```python
from build123d import *

# Parameters (mm, degrees)
SKETCH1_W               = 25
SKETCH1_H               = 3
BOSS_EXTRUDE1_DEPTH     = 288
SKETCH2_W               = 14
SKETCH2_H               = 20
SKETCH2_W_2             = 10
SKETCH2_H_2             = 16
BOSS_EXTRUDE2_DEPTH     = 18
CUT_EXTRUDE1_DEPTH      = 290.317299863
CUT_EXTRUDE1_DEPTH_BACK = 290.317299863
SKETCH3_R               = 2.5
SKETCH4_W               = 30
SKETCH4_H               = 50
BOSS_EXTRUDE3_DEPTH     = 2
BOSS_EXTRUDE4_DEPTH     = 7
FILLET1_R               = 1
SKETCH6_R               = 2.5
CUT_EXTRUDE2_DEPTH      = 10


with BuildPart() as part:
    # Sketch1 → Boss-Extrude1 (new body)
    with BuildSketch(Plane(origin=(0, 0, 0), x_dir=(1, 0, 0), z_dir=(0, 1, 0))):
        Rectangle(SKETCH1_W, SKETCH1_H)
    extrude(amount=BOSS_EXTRUDE1_DEPTH)

    # Sketch2 → Boss-Extrude2 (add)
    with BuildSketch(Plane.XY.offset(1.5)):
        with Locations((0, 278)):
            Rectangle(SKETCH2_W, SKETCH2_H)
        with Locations((0, 278)):
            Rectangle(SKETCH2_W_2, SKETCH2_H_2, mode=Mode.SUBTRACT)
    extrude(amount=BOSS_EXTRUDE2_DEPTH)

    # Sketch3 → Cut-Extrude1 (cut, two sides: drawn at the far end of the back side and taken through both)
    with BuildSketch(Plane.ZY.offset(7).offset(-CUT_EXTRUDE1_DEPTH_BACK)):
        with Locations(Location((6.5, 278, 0), (0, 0, 180))):
            Circle(SKETCH3_R)
    extrude(amount=CUT_EXTRUDE1_DEPTH + CUT_EXTRUDE1_DEPTH_BACK, mode=Mode.SUBTRACT)

    # Sketch4 → Boss-Extrude3 (add)
    with BuildSketch(Plane(origin=(0, 0, 0), x_dir=(-1, 0, 0), z_dir=(0, -1, 0))):
        Rectangle(SKETCH4_W, SKETCH4_H)
    extrude(amount=BOSS_EXTRUDE3_DEPTH)

    # Sketch5 → Boss-Extrude4 (add)
    with BuildSketch(Plane.XY.offset(1.5)):
        Polygon((0, 0), (1, 0), (1, 268), (0, 268), (-1, 268), (-1, 0), align=None)
    extrude(amount=BOSS_EXTRUDE4_DEPTH)

    # Fillet1
    fillet1_edges = [part.edges().sort_by_distance(p)[0] for p in [
        (-12.5, 288, 0),
        (9.75, 288, 1.5),
        (-9.75, 288, 1.5),
        (7, 278, 19.5),
        (0, 288, 19.5),
        (-7, 278, 19.5),
        (0, 268, 19.5),
        (7, 278, 1.5),
        (7, 268, 10.5),
        (7, 288, 10.5),
        (-7, 278, 1.5),
        (-7, 288, 10.5),
        (-4, 268, 1.5),
        (-7, 268, 10.5),
        (4, 268, 1.5),
        (1, 134, 1.5),
        (1, 268, 5),
        (-1, 134, 1.5),
        (-1, 268, 5),
        (1, 134, 8.5),
        (0, 268, 8.5),
        (-1, 134, 8.5),
        (0, 288, -1.5),
    ]]
    fillet(fillet1_edges, radius=FILLET1_R - 0.0001)  # a hair under: the kernel refuses the full size

    # Sketch6 → Cut-Extrude2 (cut)
    with BuildSketch(Plane(origin=(0, 0, 0), x_dir=(1, 0, 0), z_dir=(0, 1, 0))):
        with Locations(Location((8, 18, 0), (0, 0, 270))):
            Circle(SKETCH6_R)
        with Locations(Location((-8, 18, 0), (0, 0, 270))):
            Circle(SKETCH6_R)
        with Locations(Location((-8, -18, 0), (0, 0, 270))):
            Circle(SKETCH6_R)
        with Locations(Location((8, -18, 0), (0, 0, 270))):
            Circle(SKETCH6_R)
    extrude(amount=-CUT_EXTRUDE2_DEPTH, mode=Mode.SUBTRACT)


solid = part.part
```
The model under review builds one solid part; all positions refer to its coordinate system, in mm. A direction names the side the tool comes from. Give positions to 0.01 mm unless a question says otherwise; leave off trailing zeros. Write each loop counter-clockwise with the first axis right and the second up, starting at its lowest first coordinate (ties: lowest second). Pieces come first, ordered by that corner, then holes. Notation, with made-up numbers: M -11,16 L -5,16 A19 ccw -5,41 Z; hole C 51.25,7.5 d3. An arc over 180 degrees is marked long. Answer in a Markdown table with one row per item.
Item 1: Add section A-A on z = -18. Give the boundary of the cut face in (x, y), plus the area to 3 significant figures.
Check sheet entries:
| item | result |
|---|---|
| outline | M -15,-2 L -10.5,-2 L -10.5,0 L -15,0 Z; M -5.5,-2 L 5.5,-2 L 5.5,0 L -5.5,0 Z; M 10.5,-2 L 15,-2 L 15,0 L 10.5,0 Z |
| area | 40.0 mm2 |
Item 2: Add section B-B on y = 278. Give the boundary of the cut face in (x, z), plus the area to 3 significant figures.
Check sheet entries:
| item | result |
|---|---|
| outline | M -12.5,-1.5 L 12.5,-1.5 L 12.5,1.5 L 8,1.5 A1 cw 7,2.5 L 7,4 L 5,4 L 5,1.5 L -5,1.5 L -5,4 L -7,4 L -7,2.5 A1 cw -8,1.5 L -12.5,1.5 Z; M -7,9 L -5,9 L -5,19.5 L -6,19.5 A1 ccw -7,18.5 Z; M 5,9 L 7,9 L 7,18.5 A1 ccw 6,19.5 L 5,19.5 Z |
| area | 127 mm2 |
Item 3: For P1, Ø6, axis at x = 0, y = 274, coming from the +Z side; P2, Ø1.5, axis at x = -2, z = -9.5, coming from the +Y side; P3, Ø6.5, axis at x = -8, z = 18, coming from the -Y side; P4, Ø6.5, axis at y = 278, z = 6.5, coming from the +X side, all flat-tipped, find the tip position at first contact; note any pin that passes through.
Check sheet entries:
| item | result |
|---|---|
| P1 | z = 1.5 |
| P2 | y = 0 |
| P3 | y = -2 |
| P4 | x = 7 |
Item 4: For line 1 along X through (y, z) = (-1.2, -18); line 2 along Y through (x, z) = (-5.6, 6.5); line 3 along Y through (x, z) = (0.5, 15), list the stretches that pass through material, from the lowest coordinate up.
Check sheet entries:
| item | result |
|---|---|
| line 1 | -15 to -10.5, -5.5 to 5.5, 10.5 to 15 |
| line 2 | -2 to 0, 268 to 275.5, 280.5 to 288 |
| line 3 | -2 to 0, 268 to 270, 286 to 288 |
Item 5: Tool access review of faces 1 (the face through (0, 278, 1.5)), 2 (the face through (1, 132, 5)), 3 (the face through (0, 141, -1.5)), 4 (the face through (6.5, -1, 16)), 5 (the face through (-5.4, 278.7, 19.5)): name each direction out of +Z, -Z, +X, -X, +Y, -Y from which nothing blocks a thin tool from reaching the whole face with its end or side.
Check sheet entries:
| item | result |
|---|---|
| face 1 | +Z |
| face 2 | +Z, +X |
| face 3 | -Z, +X, -X, +Y |
| face 4 | -Y |
| face 5 | +Z, +X, -X, +Y |
Item 6: Draft analysis for pull direction Y (two halves, no side actions). For faces 6 (the face through (0, -2, 0)), 7 (the face through (0, 268, 10)), 8 (the face through (7, 141, 1.5)), 9 (the face through (6.5, -1, -20)), state which applies: +Y half, -Y half, draft (parallel to the pull), parting line (faces both ways), or undercut.
Check sheet entries:
| item | result |
|---|---|
| face 6 | -Y half |
| face 7 | undercut |
| face 8 | undercut |
| face 9 | draft |
